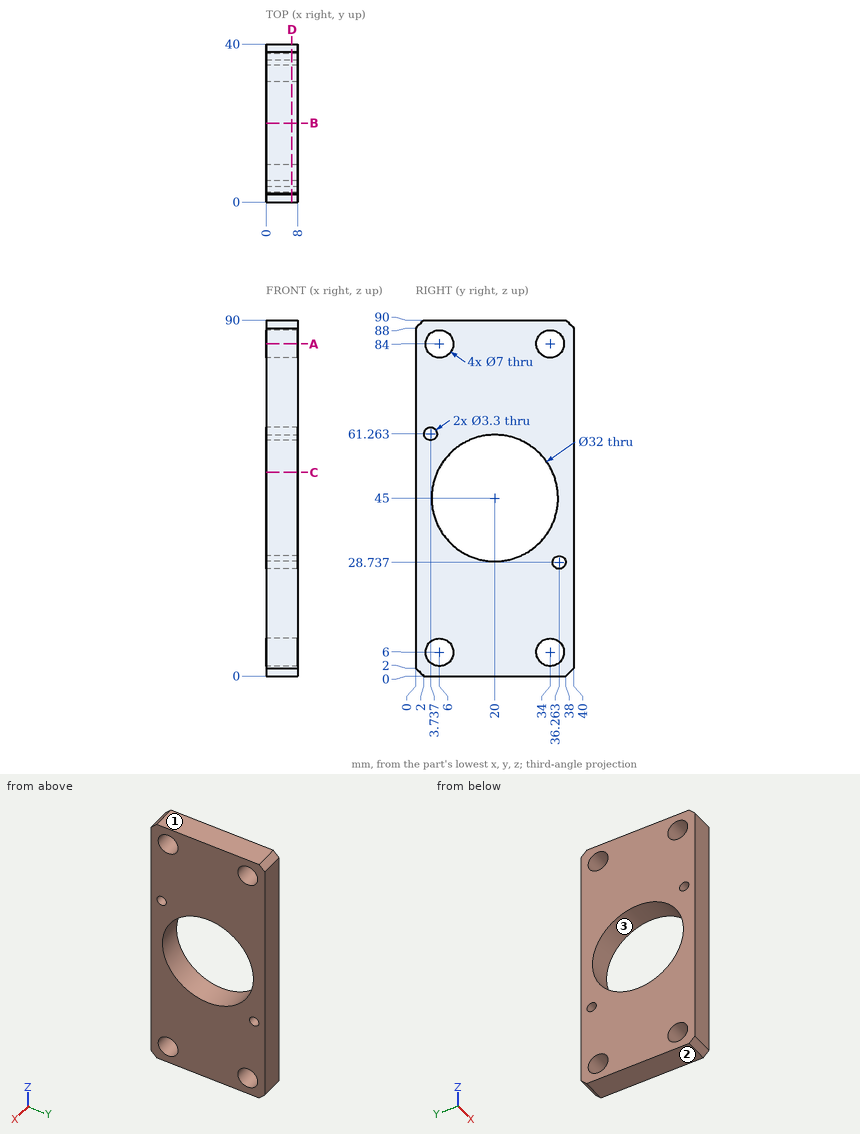
Print and shaded views of the part. All mm, measured from the part's lowest x, y and z. Round coordinates to 2 decimals unless told otherwise and drop trailing zeros. Write each loop counter-clockwise with the first axis right and the second up, starting at its lowest first coordinate (ties: lowest second). Pieces come first, ordered by that corner, then holes. Notation, with made-up numbers: (44, 54) -> (95, 54) arc R19 cw to (95, 78) -> close; hole circle Ø6 at (-5, -21). An arc over 180 degrees is marked (long way). Return JSON: item names as keys, results as strings. Group by question number.
Q1. Probe L1, parallel to Y at x = 5, z = 84; L2, parallel to Z at x = 1, y = 33 (1 decimal); L3, parallel to Z at x = 4.25, y = 32 (1 decimal). List the from-to ranges inside material, lowest first. Write a range as [from, to].
Q2. Saw through at C-C on z = 51.5. Write the cut outline in (x, y).
Q3. Saw through at A-A on z = 84. Write the cut outline in (x, y).
Q4. Saw through at B-B on y = 20. Write the cut outline in (x, z), plus the area to 3 significant figures.
Q5. Mould opens along Z. For the marked faces 1, 2 and 3 say: pulls with the +Z half, pulls with the -Z half, needs draft (parallel to the pull), parting line crosses it, or undercut.
Q6. Saw through at D-D on x = 6.5. Write the cut outline in (y, z), plus the area to 3 significant figures.
Answer:
{
 "1": {"L1": "[0, 2.5], [9.5, 30.5], [37.5, 40]", "L2": "[0, 2.6], [9.4, 35.7], [54.3, 80.6], [87.4, 90]", "L3": "[0, 3.1], [8.9, 34.4], [55.6, 81.1], [86.9, 90]"},
 "2": {"outline": "(0, 0) -> (8, 0) -> (8, 5.38) -> (0, 5.38) -> close; (0, 34.62) -> (8, 34.62) -> (8, 40) -> (0, 40) -> close"},
 "3": {"outline": "(0, 0) -> (8, 0) -> (8, 2.5) -> (0, 2.5) -> close; (0, 9.5) -> (8, 9.5) -> (8, 30.5) -> (0, 30.5) -> close; (0, 37.5) -> (8, 37.5) -> (8, 40) -> (0, 40) -> close"},
 "4": {"outline": "(0, 0) -> (8, 0) -> (8, 29) -> (0, 29) -> close; (0, 61) -> (8, 61) -> (8, 90) -> (0, 90) -> close", "area": "464 mm2"},
 "5": {"face 1": "pulls with the +Z half", "face 2": "pulls with the -Z half", "face 3": "undercut"},
 "6": {"outline": "(0, 2) -> (2, 0) -> (38, 0) -> (40, 2) -> (40, 88) -> (38, 90) -> (2, 90) -> (0, 88) -> close; hole circle Ø3.3 at (3.74, 61.26); hole circle Ø7 at (6, 6); hole circle Ø7 at (6, 84); hole circle Ø32 at (20, 45); hole circle Ø7 at (34, 6); hole circle Ø7 at (34, 84); hole circle Ø3.3 at (36.26, 28.74)", "area": "2,620 mm2"}
}
